Source: CAD feature listing. Evaluate the final solid. Frame: model axes, mm. A direction names the side the tool comes from. Round coordinates to 2 decimals unless told otherwise and drop trailing zeros. Order: outer loops, then holes, each group sorted by start corner. A loop starts at its lowest first (then second) coordinate and runs counter-clockwise, first axis right, second up. Notation, with made-up numbers: (-4, 59.25) -> (19, 59.25) arc R25 ccw to (19, 92.25) -> close; hole circle Ø6 at (57.25, 29.25). An arc over 180 degrees is marked (long way). Use a Markdown table: item, result. Add a question column.
```python
from build123d import *

# Parameters (mm, degrees)
LINK_SKETCH_R       = 3.25
LINK_SKETCH_R_2     = 1
LINK_EXTRUDE_DEPTH  = 4
JOINT_START         = 3.4
SKETCH1_3_R         = 3.25
SKETCH1_3_R_2       = 1
JOINT_EXTRUDE_DEPTH = 3.4


with BuildPart() as part:
    # Link Sketch → Link Extrude (new body)
    # profile 1 of 2: a face of its own
    with BuildSketch(Plane.XY):
        with BuildLine():
            Line((23.355762114, -19.54663337), (-2.625, -4.54663337))
            ThreePointArc((-2.625, -4.54663337), (-4.54663337, 2.625), (2.625, 4.54663337))
            Line((2.625, 4.54663337), (28.605762114, -10.45336663))
            ThreePointArc((28.605762114, -10.45336663), (30.527395483, -17.625), (23.355762114, -19.54663337))
        make_face()
        with Locations((25.980762114, -15)):
            Circle(LINK_SKETCH_R, mode=Mode.SUBTRACT)
        with Locations((-1.4, 0)):
            Circle(LINK_SKETCH_R_2, mode=Mode.SUBTRACT)
        with Locations((1.4, 0)):
            Circle(LINK_SKETCH_R_2, mode=Mode.SUBTRACT)
    # profile 2 of 2: a face of its own
    with BuildSketch(Plane.XY):
        with Locations((25.980762114, -15)):
            Circle(LINK_SKETCH_R)
        with Locations((24.768326548, -14.3)):
            Circle(LINK_SKETCH_R_2, mode=Mode.SUBTRACT)
        with Locations((27.193197679, -15.7)):
            Circle(LINK_SKETCH_R_2, mode=Mode.SUBTRACT)
    extrude(amount=-LINK_EXTRUDE_DEPTH)

    # Sketch1_3 → Joint Extrude (add)
    with BuildSketch(Plane.XY.offset(JOINT_START)):
        with Locations((25.980762114, -15)):
            Circle(SKETCH1_3_R)
        with Locations((24.768326548, -14.3)):
            Circle(SKETCH1_3_R_2, mode=Mode.SUBTRACT)
        with Locations((27.193197679, -15.7)):
            Circle(SKETCH1_3_R_2, mode=Mode.SUBTRACT)
    extrude(amount=-JOINT_EXTRUDE_DEPTH)


solid = part.part
```
1) Draft query along X for faces 1 (the flat face through (15.434, -2.848, -1.972)), 2 (the cylindrical face through (-4.603, 2.524, -1.972)), 3 (the cylindrical face through (25.2, -15.2, -0.2)), 4 (the flat face through (26, -15, 3.4)). Return one class per face: pulls with the +X half, pulls with the -X half, needs draft (parallel to the pull), parting line crosses it, or undercut.
2) Reachability of faces 5 (the cylindrical face through (29.08, -14.02, 1.72)), 6 (the flat face through (10.547, -12.152, -1.972)) from +Z, -Z, +X, -X, +Y, -Y: full face, straight path, thin tool, end or side. Return the list, or none.
3) Section D-D on y = -14.3. Output: boundary loops of the cut face in (x, z), then the cut area to 3 significant figures.
4) Section C-C on x = 1.4. Output: boundary loops of the cut face in (y, z).
5) First-contact query: pin 1 Ø2 at (x, z) = (20.5, 0.5) entering from +Y; pin 2 Ø3 at (y, z) = (0, 2) entering from -X; pin 3 Ø2.5 at (x, y) = (24.77, -14.3) entering from -Z; pin 4 Ø7.5 at (x, y) = (10, -3) entering from +Z. Flat tips, straight axial feed; report the tip coordinate or a pass-through.
6) Section A-A on y = 0. Output: boundary loops of the cut face in (x, z), then the cut area to 3 significant figures.
7) Line query: probe 1 along Z at (x, y) = (14, -11.25); probe 2 along Y at (x, z) = (1, -1.25); probe 3 along X at (y, z) = (-15.75, 1.75). Output: solid intervals per line, ascending. Write a range as from..to.
8) Section B-B on z = -1.5. Output: boundary loops of the cut face in (x, y) (3 decimals), then the cut area to 3 significant figures.
Conclusion:
| question | item | result |
|---|---|---|
| 1 | face 1 | pulls with the +X half |
| 1 | face 2 | parting line crosses it |
| 1 | face 3 | undercut |
| 1 | face 4 | needs draft |
| 2 | face 5 | +Z |
| 2 | face 6 | +Z, -Z, -X, -Y |
| 3 | outline | (14.27, -4) -> (23.77, -4) -> (23.77, 3.4) -> (22.81, 3.4) -> (22.81, 0) -> (14.27, 0) -> close; (25.77, -4) -> (31.18, -4) -> (31.18, 0) -> (29.15, 0) -> (29.15, 3.4) -> (25.77, 3.4) -> close |
| 3 | area | 74.4 mm^2 |
| 4 | outline | (-6.87, -4) -> (-1, -4) -> (-1, 0) -> (-6.87, 0) -> close; (1, -4) -> (5.06, -4) -> (5.06, 0) -> (1, 0) -> close |
| 5 | pin 1 | stops at y = -5.27 |
| 5 | pin 2 | passes through |
| 5 | pin 3 | stops at z = -4 |
| 5 | pin 4 | stops at z = 0 |
| 6 | outline | (-5.25, -4) -> (-2.4, -4) -> (-2.4, 0) -> (-5.25, 0) -> close; (-0.4, -4) -> (0.4, -4) -> (0.4, 0) -> (-0.4, 0) -> close; (2.4, -4) -> (10.5, -4) -> (10.5, 0) -> (2.4, 0) -> close |
| 6 | area | 47.0 mm^2 |
| 7 | probe 1 | z = -4..0 |
| 7 | probe 2 | y = -6.64..-0.92, 0.92..5.15 |
| 7 | probe 3 | x = 22.82..26.19, 28.19..29.14 |
| 8 | outline | (-2.625, -4.547) -> (23.356, -19.547) arc R5.25 ccw to (28.606, -10.453) -> (2.625, 4.547) arc R5.25 ccw to start; hole circle Ø2 at (-1.4, 0); hole circle Ø2 at (1.4, 0); hole circle Ø2 at (24.768, -14.3); hole circle Ø2 at (27.193, -15.7) |
| 8 | area | 389 mm^2 |
